Source: CAD feature listing. Evaluate the final solid. Frame: model axes, mm. A direction names the side the tool comes from. Round coordinates to 2 decimals unless told otherwise and drop trailing zeros. Order: outer loops, then holes, each group sorted by start corner. A loop starts at its lowest first (then second) coordinate and runs counter-clockwise, first axis right, second up. Notation, with made-up numbers: (3.5, 75) - (16.5, 75) arc R29 cw to (16.5, 105) - close; hole circle Ø5 at (67.5, -15). An arc over 180 degrees is marked (long way). Return JSON: item names as keys, results as strings. Group by question number.
1) Contact query for flat-ended pins moving along their axis: P1, Ø12, axis at y = 9.5, z = 8, coming from the +X side; P2, Ø1.5, axis at y = 6.5, z = 11, coming from the +X side. Output: stop coordinate, or through.
2) Ray query, line 1 (Z direction, x = -29.5, y = -11); line 2 (Z direction, x = -2, y = -14); line 3 (X direction, y = -30, z = 21). Return the intervals inside material, ascending. Write a range as from..to.
3) Section D-D, the plane y = -23. Return loops of the section in (x, z), plus the area to 3 significant figures.
4) Section B-B, the plane y = -13. Return loops of the section in (x, z).
5) Section A-A, the plane x = -0.5. Return loops of the section in (y, z).
6) Access query for faces 1 (the flat face through (-8, -40.573, 13)), 2 (the flat face through (1, -3, 25.4)). Directions: +Z, -Z, +X, -X, +Y, -Y. A direction counts if a zero-diameter tool reaches every point of the face in a straight line with its end or side. Return the directions, or none.
7) Section C-C, the plane z = 3.5. Return loops of the section in (x, y), plus the area to 3 significant figures.
```python
from build123d import *

# Parameters (mm, degrees)
F1_DEPTH = 25.4
F2_R     = 11.286244
F3_DEPTH = 12.7
F5_DEPTH = 60.933791


with BuildPart() as f1:
    # F0 (on Top) → F1 (new body)
    with BuildSketch(Plane.XY):
        Polygon((-44.223279, 20.360047), (-44.223279, -40.572744), (30.122576, -40.572744), (26.401911, 20.360047), align=None)
    extrude(amount=F1_DEPTH)

    # F2 (on face) → F3 (join)
    with BuildSketch(Plane.XY.offset(25.4)):
        with Locations((-9.318016, -9.232202)):
            Circle(F2_R)
    extrude(amount=F3_DEPTH)

    # F4 (on face) → F5 (cut, through all)
    with BuildSketch(Plane.XZ.offset(40.572744)):
        Polygon((1.968228, 38.1), (-20.604259, 38.1), (1.968228, 25.4), align=None)
    extrude(amount=-F5_DEPTH, mode=Mode.SUBTRACT)


solid = f1.part
```
Geometry check:
{
 "1": {"P1": "x = 27.43", "P2": "x = 27.29"},
 "2": {"line 1": "0..25.4", "line 2": "0..27.63", "line 3": "-44.22..29.48"},
 "3": {"outline": "(-44.22, 0) - (29.05, 0) - (29.05, 25.4) - (-44.22, 25.4) - close", "area": "1,860 mm2"},
 "4": {"outline": "(-44.22, 0) - (28.44, 0) - (28.44, 25.4) - (1.32, 25.4) - (1.32, 25.76) - (-19.96, 37.74) - (-19.96, 25.4) - (-44.22, 25.4) - close"},
 "5": {"outline": "(-40.57, 0) - (20.36, 0) - (20.36, 25.4) - (-2.19, 25.4) - (-2.19, 26.79) - (-16.28, 26.79) - (-16.28, 25.4) - (-40.57, 25.4) - close"},
 "6": {"face 1": "+Z, -Z, +X, -X, -Y", "face 2": "+Z"},
 "7": {"outline": "(-44.22, -40.57) - (30.12, -40.57) - (26.4, 20.36) - (-44.22, 20.36) - close", "area": "4,420 mm2"}
}
